Verification items for the finished model (mm, model axes). A direction names the side the tool comes from. Coordinates: 2 decimals unless noted, no trailing zeros. Order: outer loops, then holes, each group sorted by start corner. A loop starts at its lowest first (then second) coordinate and runs counter-clockwise, first axis right, second up. Notation, with made-up numbers: (60.5, -21.5) -> (83.5, -21.5) arc R24 cw to (83.5, 1.5) -> close; hole circle Ø9 at (21, -33). An arc over 180 degrees is marked (long way). Answer as CSV lines item,"result".
```python
from build123d import *

# Parameters (mm, degrees)
STORE_SOVE_ORTA_1_START = 182.5
STORE_SOVE_ORTA_1_DEPTH = 1427.5


with BuildPart() as part:
    # Sketch1 → STORE_sove_orta_1 (new body)
    with BuildSketch(Plane(origin=(0, 0, 0), x_dir=(1, 0, 0), z_dir=(0, 1, 0)).offset(STORE_SOVE_ORTA_1_START)):
        Polygon((690, -40), (690, -38.5), (701.25, -38.5), (701.25, 0), (702.75, 0), (702.75, -38.5), (714, -38.5), (714, -40), align=None)
    extrude(amount=STORE_SOVE_ORTA_1_DEPTH)


solid = part.part
```
Item 1: Thickness scan on line 1 (X direction, y = 670.5, z = 19.5); line 2 (Z direction, x = 697, y = 1310.5). Record the ranges inside material, lowest first.
Answer list:
line 1,"701.25 to 702.75"
line 2,"38.5 to 40"
Item 2: Depth check by flat-ended pin: pin 1 Ø6 at (x, z) = (708.5, 21) entering from +Y; pin 2 Ø4 at (x, y) = (710, 339.5) entering from -Z; pin 3 Ø19 at (y, z) = (980, 14.5) entering from -X; pin 4 Ø1 at (y, z) = (1325, 11) entering from +X. Enter the tip coordinate at first touch or a pass-through.
Answer list:
pin 1,"through"
pin 2,"z = 38.5"
pin 3,"x = 701.25"
pin 4,"x = 702.75"
Item 3: Section check B-B, the plane x = 708.25. Record the boundary of the cut face in (y, z), plus the area to 3 significant figures.
Answer list:
outline,"(182.5, 38.5) -> (1610, 38.5) -> (1610, 40) -> (182.5, 40) -> close"
area,"2,140 mm2"
Item 4: Section check C-C, the plane z = 25. Record the boundary of the cut face in (x, y).
Answer list:
outline,"(701.25, 182.5) -> (702.75, 182.5) -> (702.75, 1610) -> (701.25, 1610) -> close"
Item 5: Section check A-A, the plane y = 533.5. Record the boundary of the cut face in (x, z).
Answer list:
outline,"(690, 38.5) -> (701.25, 38.5) -> (701.25, 0) -> (702.75, 0) -> (702.75, 38.5) -> (714, 38.5) -> (714, 40) -> (690, 40) -> close"
Item 6: Tool access check on faces 1 (the flat face through (702, 182.5, 29)), 2 (the flat face through (701.25, 886, 20)), 3 (the flat face through (702.75, 886, 19)). Record the directions out of +Z, -Z, +X, -X, +Y, -Y that give a thin tool (end or side, any length) a straight path to the whole face; none if there is none.
Answer list:
face 1,"+Z, -Z, +X, -X, -Y"
face 2,"-Z, -X, +Y, -Y"
face 3,"-Z, +X, +Y, -Y"
